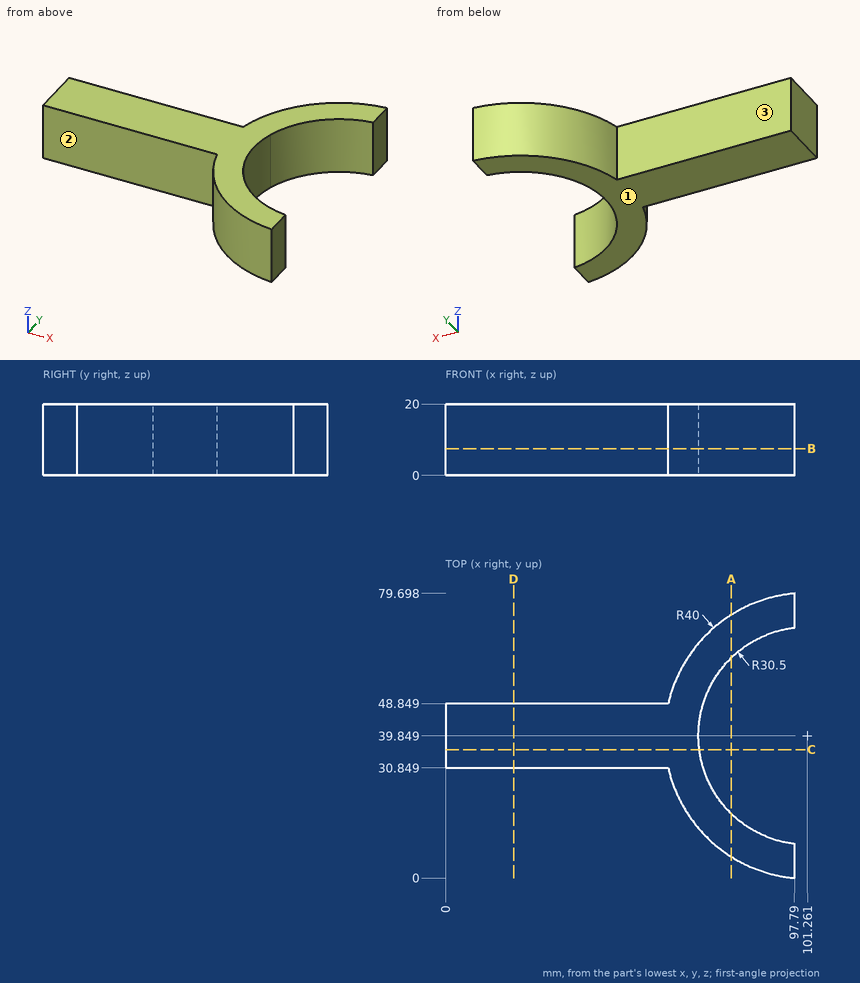
The drawing under review shows one solid part. Ordinate dimensions are in mm from its lowest x, y, z. A direction names the side the tool comes from. Give positions to 0.01 mm unless a question says otherwise; leave off trailing zeros. Loops run counter-clockwise (first coordinate to the right, second up) from the corner with the lowest first, then second, coordinate; pieces in that order, holes last. Notation, with made-up numbers: M -2,16 L 34,16 A25 cw 34,50 Z; hole C 57,-37 d6. An arc over 180 degrees is marked long. Return JSON: item names as keys, results as strings. Group by question number.
Item 1: We need section C-C (y = 36). Give the boundary of the cut face in (x, z) (1 decimal).
Item 2: Insertion check: pin 1 Ø1.5 at (x, z) = (16.5, 17.5) entering from +Y; pin 2 Ø6 at (y, z) = (62, 2) entering from +X; pin 3 Ø2 at (y, z) = (71, 4) entering from -X (1 decimal). Each pin has a flat end and moves straight along its axis. Give the tip position at first contact, or say it passes through.
Item 3: For probe 1 along Y at (x, z) = (26.5, 12.5); probe 2 along Y at (x, z) = (76, 5.75) (1 decimal); probe 3 along Y at (x, z) = (81.5, 16) (1 decimal), list the stretches that pass through material, from the lowest coordinate up.
Item 4: We need section B-B (z = 7.5). Give the boundary of the cut face in (x, y).
Item 5: Tool access review of the marked faces 1, 2 and 3: name each direction out of +Z, -Z, +X, -X, +Y, -Y from which nothing blocks a thin tool from reaching the whole face with its end or side.
Item 6: We need section D-D (x = 19). Give the boundary of the cut face in (y, z).
Item 7: We need section A-A (x = 80). Give the boundary of the cut face in (y, z).
Output:
{
 "1": {"outline": "M 0,0 L 71,0 L 71,20 L 0,20 Z"},
 "2": {"pin 1": "stops at y = 48.85", "pin 2": "stops at x = 84.01", "pin 3": "stops at x = 75"},
 "3": {"probe 1": "y = 30.85 to 48.85", "probe 2": "y = 8.8 to 22.8, 56.9 to 70.9", "probe 3": "y = 5.1 to 16.6, 63.1 to 74.6"},
 "4": {"outline": "M 0,30.85 L 62.29,30.85 A40 ccw 97.79,0 L 97.79,9.55 A30.5 cw 97.79,70.15 L 97.79,79.7 A40 ccw 62.29,48.85 L 0,48.85 Z"},
 "5": {"face 1": "-Z, +X, -X, +Y, -Y", "face 2": "+Z, -Z, -X, -Y", "face 3": "+Z, -Z, -X, +Y"},
 "6": {"outline": "M 30.85,0 L 48.85,0 L 48.85,20 L 30.85,20 Z"},
 "7": {"outline": "M 5.97,0 L 17.98,0 L 17.98,20 L 5.97,20 Z; M 61.72,0 L 73.73,0 L 73.73,20 L 61.72,20 Z"}
}
